Work out the finished part from the listing and answer in its coordinate system (mm). A direction names the side the tool comes from. Coordinates: 2 decimals unless noted, no trailing zeros. Loops run counter-clockwise (first coordinate to the right, second up) from the corner with the lowest first, then second, coordinate; pieces in that order, holes last. Notation, with made-up numbers: (-22, 69) - (2, 69) arc R20 ccw to (2, 103) - close; hole circle Ø1 at (72, -23). An arc over 180 degrees is marked (long way). Write each question's results on one line, items separated by ' | '. Start each with the question number.
1. A cutting plane is placed at B-B on x = 34.5. Determine the outline of the cut face in (y, z), then the cut area to 3 significant figures.
2. Which of the six approach directions +Z, -Z, +X, -X, +Y, -Y give full straight-line access (tool end or side, diameter ignored) to faces 1 (the flat face through (0, 51, -196)), 2 (the flat face through (3, 51, -97)), 3 (the flat face through (-3, 49, -97)), 4 (the flat face through (0, 0, -97))?
3. A cutting plane is placed at C-C on z = -8.5. Determine the outline of the cut face in (x, y).
4. A cutting plane is placed at A-A on y = 41. Determine the outline of the cut face in (x, z).
5. Find the intervals of material crossed by line 1 along Z through (x, y) = (-75.5, -44); line 2 along X through (y, z) = (87, -129), in increasing order. Write a range as [from, to].
6. Each of these flat-tipped pins is pushed along its axis until it touches: P1, Ø6, axis at x = -36.5, y = -70.5, coming from the -Z side; P2, Ø12, axis at y = 1, z = -170, coming from the +X side; P3, Ø5, axis at x = 0.5, z = -121, coming from the -Y side. Where does it stop, or does it pass through?
from build123d import *

# Parameters (mm, degrees)
SZKIC1_W                    = 100
SZKIC1_H                    = 100
DODANIE_WYCI_GNI_CIE1_DEPTH = 4
DODANIE_WYCI_GNI_CIE2_DEPTH = 196


with BuildPart() as part:
    # Szkic1 → Dodanie-wyciągnięcie1 (new body)
    with BuildSketch(Plane.XY):
        with Locations((-50, 50)):
            Rectangle(SZKIC1_W, SZKIC1_H)
        with Locations((50, 50)):
            Rectangle(SZKIC1_W, SZKIC1_H)
        with Locations((50, -50)):
            Rectangle(SZKIC1_W, SZKIC1_H)
        with Locations((-50, -50)):
            Rectangle(SZKIC1_W, SZKIC1_H)
    extrude(amount=DODANIE_WYCI_GNI_CIE1_DEPTH)

    # Szkic2 → Dodanie-wyciągnięcie2 (add)
    with BuildSketch(Plane(origin=(0, 0, 0), x_dir=(-1, 0, 0), z_dir=(0, 0, -1))):
        Polygon((0, 0), (3, 0), (3, 100), (-3, 100), (-3, 0), align=None)
    extrude(amount=DODANIE_WYCI_GNI_CIE2_DEPTH)


solid = part.part
Values:
1) outline: (-100, 0) - (100, 0) - (100, 4) - (-100, 4) - close | area: 800 mm^2
2) face 1: -Z, +X, -X, +Y, -Y | face 2: -Z, +X, +Y, -Y | face 3: -Z, -X, +Y, -Y | face 4: -Z, +X, -X, -Y
3) outline: (-3, 0) - (3, 0) - (3, 100) - (-3, 100) - close
4) outline: (-100, 0) - (-3, 0) - (-3, -196) - (3, -196) - (3, 0) - (100, 0) - (100, 4) - (-100, 4) - close
5) line 1: [0, 4] | line 2: [-3, 3]
6) P1: z = 0 | P2: x = 3 | P3: y = 0
